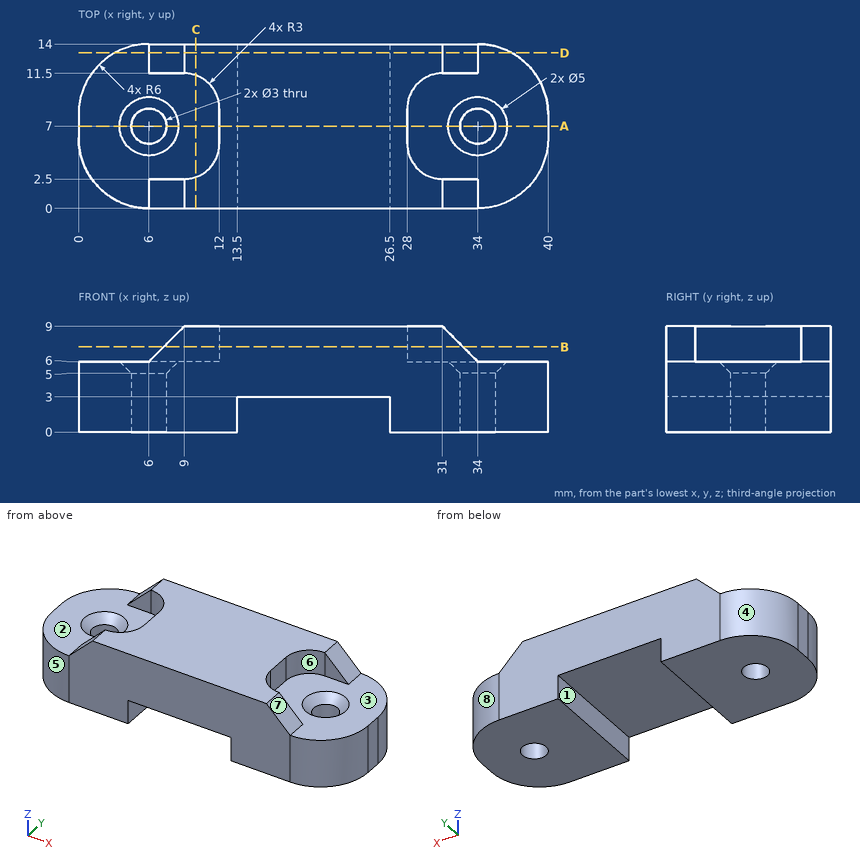
Drawing for the job (mm, zero at the part's lowest x, y, z). A direction names the side the tool comes from. Round coordinates to 2 decimals unless told otherwise and drop trailing zeros. Order: outer loops, then holes, each group sorted by start corner. A loop starts at its lowest first (then second) coordinate and runs counter-clockwise, first axis right, second up. Notation, with made-up numbers: (46, 87) -> (102, 87) arc R7 ccw to (102, 92) -> close; hole circle Ø4 at (56.5, 72.25). An arc over 180 degrees is marked (long way). Put each result on its own line as item: value.
Q1. Pull direction Y, two halves, no side cores. Call the marked faces 5, 6, 7 and 8: pulls with the +Y half, pulls with the -Y half, needs draft (parallel to the pull), parting line crosses it, or undercut.
From the geometry:
face 5: pulls with the -Y half
face 6: undercut
face 7: needs draft
face 8: pulls with the +Y half
Q2. Pin check, flat tips, straight feed: pin 1 Ø6 at (x, y) = (36, 5.5) entering from +Z; pin 2 Ø1.5 at (y, z) = (11.5, 8) entering from -X; pin 3 Ø2.5 at (x, y) = (34, 7) entering from +Z; pin 4 Ø2.5 at (y, z) = (7, 7.5) entering from -X. Stop position of each tip, or through.
From the geometry:
pin 1: stops at z = 6
pin 2: stops at x = 7.25
pin 3: passes through
pin 4: stops at x = 12
Q3. Wall check: line 1 (X direction, y = 7, z = 3.75); line 2 (Y direction, x = 6, z = 3.7); line 3 (X direction, y = 6.5, z = 1.75). Give the ranges that are in metal, low to high. Write a range as [from, to].
From the geometry:
line 1: x = [0, 4.5], [7.5, 32.5], [35.5, 40]
line 2: y = [0, 5.5], [8.5, 14]
line 3: x = [0, 4.59], [7.41, 13.5], [26.5, 32.59], [35.41, 40]
Q4. Band-saw the part on D-D (y = 13.25). Give the cut face in (x, z).
From the geometry:
outline: (3.1, 0) -> (13.5, 0) -> (13.5, 3) -> (26.5, 3) -> (26.5, 0) -> (36.9, 0) -> (36.9, 6) -> (34, 6) -> (31, 9) -> (9, 9) -> (6, 6) -> (3.1, 6) -> close
Q5. Band-saw the part on C-C (x = 10). Give the cut face in (y, z).
From the geometry:
outline: (0, 0) -> (14, 0) -> (14, 9) -> (11.33, 9) -> (11.33, 6) -> (2.67, 6) -> (2.67, 9) -> (0, 9) -> close
Q6. Band-saw the part on A-A (y = 7). Give the cut face in (x, z).
From the geometry:
outline: (0, 0) -> (4.5, 0) -> (4.5, 5) -> (3.5, 6) -> (0, 6) -> close; (7.5, 0) -> (13.5, 0) -> (13.5, 3) -> (26.5, 3) -> (26.5, 0) -> (32.5, 0) -> (32.5, 5) -> (31.5, 6) -> (28, 6) -> (28, 9) -> (12, 9) -> (12, 6) -> (8.5, 6) -> (7.5, 5) -> close; (35.5, 0) -> (40, 0) -> (40, 6) -> (36.5, 6) -> (35.5, 5) -> close
Q7. Band-saw the part on B-B (z = 7.25). Give the cut face in (x, y), and give its area (3 significant figures).
From the geometry:
outline: (7.25, 0) -> (32.75, 0) -> (32.75, 2.5) -> (31, 2.5) arc R3 cw to (28, 5.5) -> (28, 8.5) arc R3 cw to (31, 11.5) -> (32.75, 11.5) -> (32.75, 14) -> (7.25, 14) -> (7.25, 11.5) -> (9, 11.5) arc R3 cw to (12, 8.5) -> (12, 5.5) arc R3 cw to (9, 2.5) -> (7.25, 2.5) -> close
area: 279 mm2
Q8. Tool access for the marked faces 1, 2, 3 and 4: list every direction of +Z, -Z, +X, -X, +Y, -Y with a clear straight run to the whole face (end or side of a thin tool).
From the geometry:
face 1: -Z, +Y, -Y
face 2: +Z, -X
face 3: +Z, +X
face 4: +Z, -Z, -X, +Y
